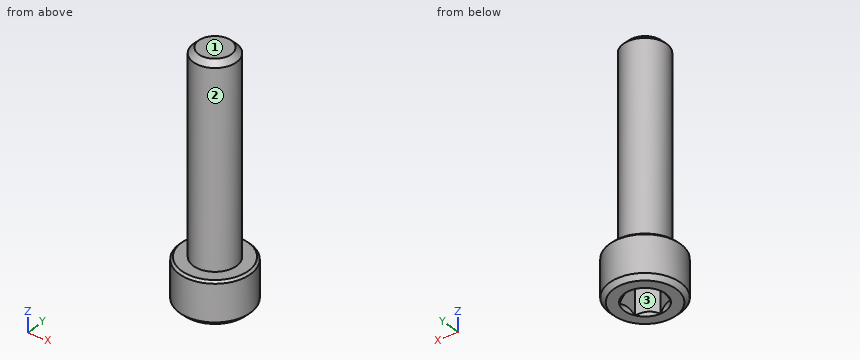
from build123d import *

# Parameters (mm, degrees)
SKETCH1_R          = 2.413
EXTRUDE1_DEPTH     = 22.225
CHAMFER3_SIZE      = 0.5953125
SKETCH6_R          = 3.9624
EXTRUDE2_DEPTH     = 4.826
CUT_EXTRUDE1_DEPTH = 2.9765625
SKETCH8_R          = 2.291358881
CUT_EXTRUDE2_DEPTH = 0.4826
CUT_EXTRUDE2_DRAFT = -45
CHAMFER1_SIZE      = 0.4826
CHAMFER2_SIZE      = 0.2413


with BuildPart() as part:
    # Sketch1 → Extrude1 (new body)
    with BuildSketch(Plane.XY):
        Circle(SKETCH1_R)
    extrude(amount=-EXTRUDE1_DEPTH)

    # Chamfer3
    chamfer3_edges = [part.edges().sort_by_distance(p)[0] for p in [
        (-2.413, 0, 0),
    ]]
    chamfer(chamfer3_edges, length=CHAMFER3_SIZE)

    # Sketch6 → Extrude2 (add)
    with BuildSketch(Plane(origin=(0, 0, -22.225), x_dir=(-1, 0, 0), z_dir=(0, 0, -1))):
        Circle(SKETCH6_R)
    extrude(amount=EXTRUDE2_DEPTH)

    # Sketch7 → Cut-Extrude1 (cut)
    with BuildSketch(Plane(origin=(0, 0, -27.051), x_dir=(-1, 0, 0), z_dir=(0, 0, -1))):
        Polygon((0, 2.291358881), (-1.984375, 1.14567944), (-1.984375, -1.14567944), (0, -2.291358881), (1.984375, -1.14567944), (1.984375, 1.14567944), align=None)
    extrude(amount=-CUT_EXTRUDE1_DEPTH, mode=Mode.SUBTRACT)


with BuildPart() as cut_extrude2_tool:
    # Sketch8 → Cut-Extrude2 (with draft: the straight prism first)
    with BuildSketch(Plane(origin=(0, 0, -27.051), x_dir=(-1, 0, 0), z_dir=(0, 0, -1))):
        Circle(SKETCH8_R)
    extrude(amount=-CUT_EXTRUDE2_DEPTH)
    # Cut-Extrude2: the draft: its side faces are tilted about the plane it starts from
    cut_extrude2_sides = [cut_extrude2_tool.faces().sort_by_distance(p)[0] for p in [
        (2.291358881, 0, -26.8097),
    ]]
    draft(cut_extrude2_sides, Plane(origin=(0, 0, -27.051), x_dir=(-1, 0, 0), z_dir=(0, 0, -1)), CUT_EXTRUDE2_DRAFT)


with BuildPart() as part_1:
    add(part.part)

    # Cut-Extrude2: cut by cut_extrude2_tool
    add(cut_extrude2_tool.part, mode=Mode.SUBTRACT)

    # Chamfer1
    chamfer1_edges = [part_1.edges().sort_by_distance(p)[0] for p in [
        (3.9624, 0, -27.051),
    ]]
    chamfer(chamfer1_edges, length=CHAMFER1_SIZE)

    # Chamfer2
    chamfer2_edges = [part_1.edges().sort_by_distance(p)[0] for p in [
        (3.9624, 0, -22.225),
    ]]
    chamfer(chamfer2_edges, length=CHAMFER2_SIZE)


solid = part_1.part
Geometry check sheet. Reference: the model listing, model coordinates, mm. Face numbers are marked on the shaded views. Round coordinates to 2 decimals unless told otherwise and drop trailing zeros. Order: outer loops, then holes, each group sorted by start corner. A loop starts at its lowest first (then second) coordinate and runs counter-clockwise, first axis right, second up. Notation, with made-up numbers: M 76.25,33.25 L 102.25,33.25 A20 ccw 102.25,69.25 Z; hole C 9,-28 d4. An arc over 180 degrees is marked long. Answer in a Markdown table with one row per item.
(1) Go/stop test with flat-tipped pins: P1, Ø1, axis at x = 1.5, z = -13.5, coming from the -Y side; P2, Ø3, axis at y = -1, z = -20.5, coming from the +X side; P3, Ø3, axis at x = 2.5, z = -12, coming from the +Y side. Record where each tip stops, or that it passes through.
Responses:
| item | result |
|---|---|
| P1 | stops at y = -2.2 |
| P2 | stops at x = 2.41 |
| P3 | stops at y = 2.2 |
(2) Sectioned sample at B-B, the plane y = 0. Record the cut outline in (x, z) (3 decimals).
Responses:
| item | result |
|---|---|
| outline | M -3.962,-26.568 L -3.48,-27.051 L -2.291,-27.051 L -1.984,-26.744 L -1.984,-24.074 L 1.984,-24.074 L 1.984,-26.744 L 2.291,-27.051 L 3.48,-27.051 L 3.962,-26.568 L 3.962,-22.466 L 3.721,-22.225 L 2.413,-22.225 L 2.413,-0.595 L 1.818,0 L -1.818,0 L -2.413,-0.595 L -2.413,-22.225 L -3.721,-22.225 L -3.962,-22.466 Z |
(3) Sectioned sample at A-A, the plane z = -25. Record the cut outline in (x, y), and give its area (3 significant figures).
Responses:
| item | result |
|---|---|
| outline | C 0,0 d7.92; hole M -1.98,-1.15 L 0,-2.29 L 1.98,-1.15 L 1.98,1.15 L 0,2.29 L -1.98,1.15 Z |
| area | 35.7 mm² |
(4) Scan lines: probe 1 along Y at (x, z) = (0.75, -3.75); probe 2 along Y at (x, z) = (1.5, -25.25); probe 3 along Z at (x, y) = (-0.5, 0.5). Record each from-to range of solid material in increasing order. Write a range as from..to.
Responses:
| item | result |
|---|---|
| probe 1 | y = -2.29..2.29 |
| probe 2 | y = -3.67..-1.43, 1.43..3.67 |
| probe 3 | z = -24.07..0 |
(5) Draft check along X on the marked faces 1, 2 and 3. Enter one of: released by +X, released by -X, zero draft, split by the parting line, or undercut.
Responses:
| item | result |
|---|---|
| face 1 | zero draft |
| face 2 | split by the parting line |
| face 3 | undercut |
(6) Sectioned sample at C-C, the plane z = -20.5. Record the cut outline in (x, y), and give its area (3 significant figures).
Responses:
| item | result |
|---|---|
| outline | C 0,0 d4.83 |
| area | 18.3 mm² |
